```python
from build123d import *

# Parameters (mm, degrees)
SKETCH2_W = 1.5
SKETCH2_H = 6


with BuildPart() as part:
    # Sweep1: sweep along a path in Sketch1
    with BuildLine(Plane.XY) as sweep1_path:
        Line((-42.529793069, 385.761298089), (-8.716710208, -0.762537307))
        ThreePointArc((-8.716710208, -0.762537307), (0.816439483, -8.711826822), (8.706610119, 0.870310423))
        Line((8.706610119, 0.870310423), (-29.885440603, 386.946279013))
        ThreePointArc((-29.885440603, 386.946279013), (-36.796453743, 392.636979485), (-42.529793069, 385.761298089))
    # Sketch2 → Sweep1 (sweep)
    with BuildSketch(Plane(origin=(-25.623251639, 192.499380391, 0), x_dir=(-0.996195452, -0.087147121, 0), z_dir=(0.087147121, -0.996195452, 0))):
        with Locations((0.75, 0)):
            Rectangle(SKETCH2_W, SKETCH2_H)
    sweep(path=sweep1_path.line)


solid = part.part
```
The model under review builds one solid part; all positions refer to its coordinate system, in mm. A direction names the side the tool comes from. Give positions to 0.01 mm unless a question says otherwise; leave off trailing zeros. Write each loop counter-clockwise with the first axis right and the second up, starting at its lowest first coordinate (ties: lowest second). Pieces come first, ordered by that corner, then holes. Notation, with made-up numbers: M 1.25,2.5 L 13.25,2.5 A27 cw 13.25,27.5 Z; hole C 75.5,30.5 d11. An arc over 180 degrees is marked long. Answer in a Markdown table with one row per item.
Item 1: Draft analysis for pull direction X (two halves, no side actions). For faces 1 (the face through (0.62, -8.73, 0.04)), 2 (the face through (-26, 190, 3)), 3 (the face through (0.731, -10.224, -0.042)), state which applies: +X half, -X half, draft (parallel to the pull), parting line (faces both ways), or undercut.
Check sheet entries:
| item | result |
|---|---|
| face 1 | undercut |
| face 2 | draft |
| face 3 | parting line |
Item 2: For P1, Ø2, axis at y = 147.5, z = 0, coming from the -X side; P2, Ø2, axis at x = -22, y = 336, coming from the -Z side; P3, Ø1, axis at y = 179, z = -1.5, coming from the +X side, all flat-tipped, find the tip position at first contact; note any pin that passes through.
Check sheet entries:
| item | result |
|---|---|
| P1 | x = -23.28 |
| P2 | through |
| P3 | x = -7.54 |
Item 3: Add section C-C on y = 357. Give the boundary of the cut face in (x, z), plus the area to 3 significant figures.
Check sheet entries:
| item | result |
|---|---|
| outline | M -41.52,-3 L -40.01,-3 L -40.01,3 L -41.52,3 Z; M -26.89,-3 L -25.38,-3 L -25.38,3 L -26.89,3 Z |
| area | 18.1 mm2 |
Item 4: Add section B-B on x = 0. Give the boundary of the cut face in (y, z), plus the area to 3 significant figures.
Check sheet entries:
| item | result |
|---|---|
| outline | M -10.25,-3 L -8.75,-3 L -8.75,3 L -10.25,3 Z; M 87.97,-3 L 103.05,-3 L 103.05,3 L 87.97,3 Z |
| area | 99.5 mm2 |
Item 5: Tool access review of faces 4 (the face through (-9.367, 196.76, 0.042)), 5 (the face through (-36.66, 392.65, 0.04)): name each direction out of +Z, -Z, +X, -X, +Y, -Y from which nothing blocks a thin tool from reaching the whole face with its end or side.
Check sheet entries:
| item | result |
|---|---|
| face 4 | +Z, -Z, +X, +Y |
| face 5 | +Z, -Z |
Item 6: For line 1 along X through (y, z) = (233, 0.5); line 2 along X through (y, z) = (129.5, 0.75), list the stretches that pass through material, from the lowest coordinate up.
Check sheet entries:
| item | result |
|---|---|
| line 1 | -30.67 to -29.17, -14.5 to -12.99 |
| line 2 | -21.62 to -20.11, -4.15 to -2.64 |
Item 7: Add section A-A on z = -1.5. Give the boundary of the cut face in (x, y).
Check sheet entries:
| item | result |
|---|---|
| outline | M -44.02,385.63 L -10.21,-0.89 A10.25 ccw long 10.2,1.02 L -28.39,387.1 A7.85 ccw Z; hole M -42.53,385.76 L -8.72,-0.76 A8.75 ccw long 8.71,0.87 L -29.89,386.95 A6.35 ccw Z |
